Drawing for the job (mm, zero at the part's lowest x, y, z). Coordinates: 2 decimals unless noted, no trailing zeros. One line per item, written item: value.
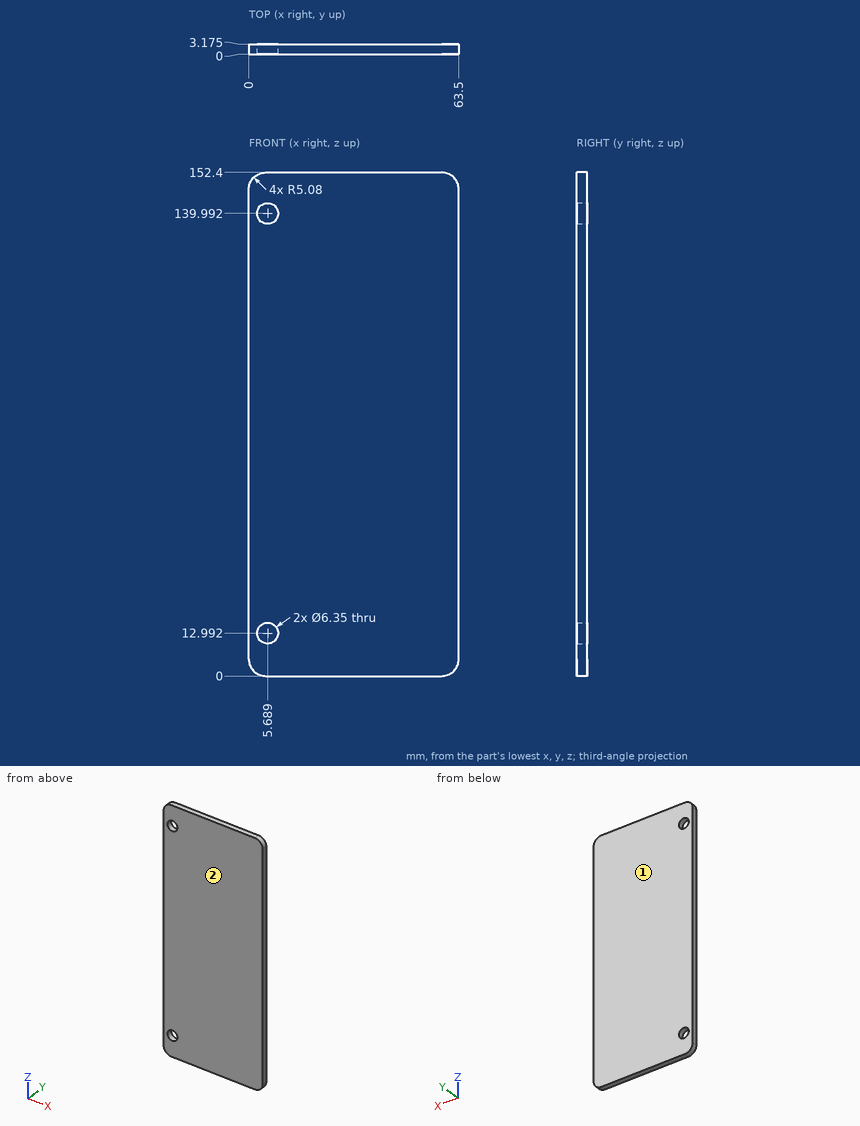
Item 1: Probe probe 1 along Z at (x, y) = (7.5, 0.9) (1 decimal); probe 2 along X at (y, z) = (2.65, 142); probe 3 along Z at (x, y) = (61.5, 0.4). List the from-to ranges inside material, lowest first. Write a range as from..to.
Check result:
probe 1: z = 0..10.4, 15.6..137.4, 142.6..152.4
probe 2: x = 0..3.23, 8.15..63.5
probe 3: z = 1.04..151.36
Item 2: Drop a flat-ended pin along its axis: P1, Ø4, axis at x = 5.69, z = 12.99, coming from the +Y side. Give the stop position or say it passes through.
Check result:
P1: passes through
Item 3: Pull direction Y, two halves, no side cores. Call the marked faces 1 and 2: released by +Y, released by -Y, zero draft, split by the parting line, or undercut.
Check result:
face 1: released by +Y
face 2: released by -Y
